Here's how the part is built. I have some questions about the finished solid (model axes, mm). Face numbers are marked on the shaded views. A direction names the side the tool comes from. Coordinates: 2 decimals unless noted, no trailing zeros. Loops run counter-clockwise (first coordinate to the right, second up) from the corner with the lowest first, then second, coordinate; pieces in that order, holes last. Notation, with made-up numbers: (47, -22.5) - (56, -22.5) arc R15 cw to (56, 1.5) - close; hole circle Ø8 at (66, 8). An arc over 180 degrees is marked (long way). Use a Markdown table: item, result.
```python
from build123d import *

# Parameters (mm, degrees)
BOSS_EXTRUDE1_DEPTH            = 50
SKETCH2_R                      = 8.75
SKETCH2_R_2                    = 2.1
CUT_EXTRUDE1_DEPTH             = 10
FILLET1_R                      = 2
FILLET2_R                      = 0.5
FILLET3_R                      = 0.5
HOLE_FOR_M4_300_SC_NUTS_SP_1_D = 4


with BuildPart() as part:
    # Sketch1 → Boss-Extrude1 (new body)
    with BuildSketch(Plane.XY):
        with BuildLine():
            Line((0, 0), (0, 49))
            Line((0, 49), (-3, 49))
            Line((-3, 49), (-3, -2))
            ThreePointArc((-3, -2), (-2.707106781, -2.707106781), (-2, -3))
            Line((-2, -3), (49, -3))
            Line((49, -3), (49, 0))
            Line((49, 0), (0, 0))
        make_face()
    extrude(amount=BOSS_EXTRUDE1_DEPTH)

    # Sketch2 → Cut-Extrude1 (cut)
    with BuildSketch(Plane(origin=(0, 0, 0), x_dir=(0, 0, -1), z_dir=(1, 0, 0))):
        with Locations((-25, 25)):
            Circle(SKETCH2_R)
        with Locations((-10.5, 25)):
            Circle(SKETCH2_R_2)
        with Locations((-39.5, 25)):
            Circle(SKETCH2_R_2)
    extrude(amount=-CUT_EXTRUDE1_DEPTH, mode=Mode.SUBTRACT)

    # Fillet1
    fillet1_edges = [part.edges().sort_by_distance(p)[0] for p in [
        (-1.5, 49, 50),
        (-1.5, 49, 0),
    ]]
    fillet(fillet1_edges, radius=FILLET1_R)

    # Fillet2
    fillet2_edges = [part.edges().sort_by_distance(p)[0] for p in [
        (0, 0, 25),
    ]]
    fillet(fillet2_edges, radius=FILLET2_R)

    # Fillet3
    fillet3_edges = [part.edges().sort_by_distance(p)[0] for p in [
        (49, -1.5, 50),
        (49, -1.5, 0),
    ]]
    fillet(fillet3_edges, radius=FILLET3_R)

    # Hole for M4 300® SC Nuts (SP)1 (through all)
    with Locations(Plane(origin=(0, 0, 0), x_dir=(1, 0, 0), z_dir=(0, 1, 0))):
        with Locations((36, -13.5), (8, -13.5), (36, -36.5), (8, -36.5)):
            Hole(HOLE_FOR_M4_300_SC_NUTS_SP_1_D / 2)


solid = part.part
```
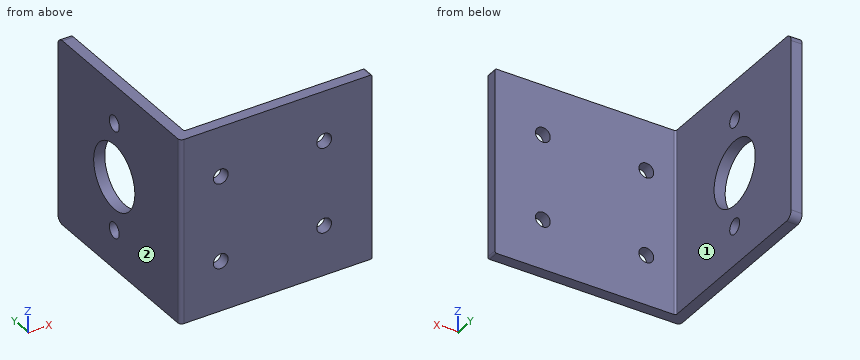
Q1. I want a section at C-C, the plane x = 36. Write out the boundary of the cut face in (y, z), then the cut area to 3 significant figures.
Check values:
| item | result |
|---|---|
| outline | (-3, 0) - (0, 0) - (0, 11.5) - (-3, 11.5) - close; (-3, 15.5) - (0, 15.5) - (0, 34.5) - (-3, 34.5) - close; (-3, 38.5) - (0, 38.5) - (0, 50) - (-3, 50) - close |
| area | 126 mm^2 |
Q2. I want a section at D-D, the plane z = 36.5. Write out the boundary of the cut face in (x, y).
Check values:
| item | result |
|---|---|
| outline | (-3, -2) arc R1 ccw to (-2, -3) - (6, -3) - (6, 0) - (0.5, 0) arc R0.5 cw to (0, 0.5) - (0, 49) - (-3, 49) - close; (10, -3) - (34, -3) - (34, 0) - (10, 0) - close; (38, -3) - (49, -3) - (49, 0) - (38, 0) - close |
Q3. I want a section at B-B, the plane y = 25. Write out the boundary of the cut face in (x, z), then the cut area to 3 significant figures.
Check values:
| item | result |
|---|---|
| outline | (-3, 0) - (0, 0) - (0, 8.4) - (-3, 8.4) - close; (-3, 12.6) - (0, 12.6) - (0, 16.25) - (-3, 16.25) - close; (-3, 33.75) - (0, 33.75) - (0, 37.4) - (-3, 37.4) - close; (-3, 41.6) - (0, 41.6) - (0, 50) - (-3, 50) - close |
| area | 72.3 mm^2 |
Q4. Which directions (+Z, -Z, +X, -X, +Y, -Y) give clear straight access to the entire face, cutting with the end or side of a thin tool? Please do the marked faces 1 and 2.
Check values:
| item | result |
|---|---|
| face 1 | +Z, -Z, +X, +Y |
| face 2 | +Z, -Z, -X, +Y, -Y |
Q5. I want a section at A-A, the plane z = 25. Write out the boundary of the cut face in (x, y), then the cut area to 3 significant figures.
Check values:
| item | result |
|---|---|
| outline | (-3, -2) arc R1 ccw to (-2, -3) - (49, -3) - (49, 0) - (0.5, 0) arc R0.5 cw to (0, 0.5) - (0, 16.25) - (-3, 16.25) - close; (-3, 33.75) - (0, 33.75) - (0, 49) - (-3, 49) - close |
| area | 250 mm^2 |
Q6. Please list where these lines run through material, in increasing order: L1, parallel to X at y = -1.2, z = 13.5; L2, parallel to Y at x = -0.65, z = 39.5; L3, parallel to Y at x = 2.5, z = 10.5. Write a range as from..to.
Check values:
| item | result |
|---|---|
| L1 | -3..6, 10..34, 38..49 |
| L2 | -3..22.9, 27.1..49 |
| L3 | -3..0 |
Q7. Will these pins go through, and if not, where does the flat tip stop? P1, Ø1.5, axis at y = 13, z = 21.5, coming from the +X side; P2, Ø3.5, axis at y = 25, z = 39.5, coming from the +X side; P3, Ø12, axis at x = 39, z = 30, coming from the +Y side.
Check values:
| item | result |
|---|---|
| P1 | x = 0 |
| P2 | through |
| P3 | y = 0 |
